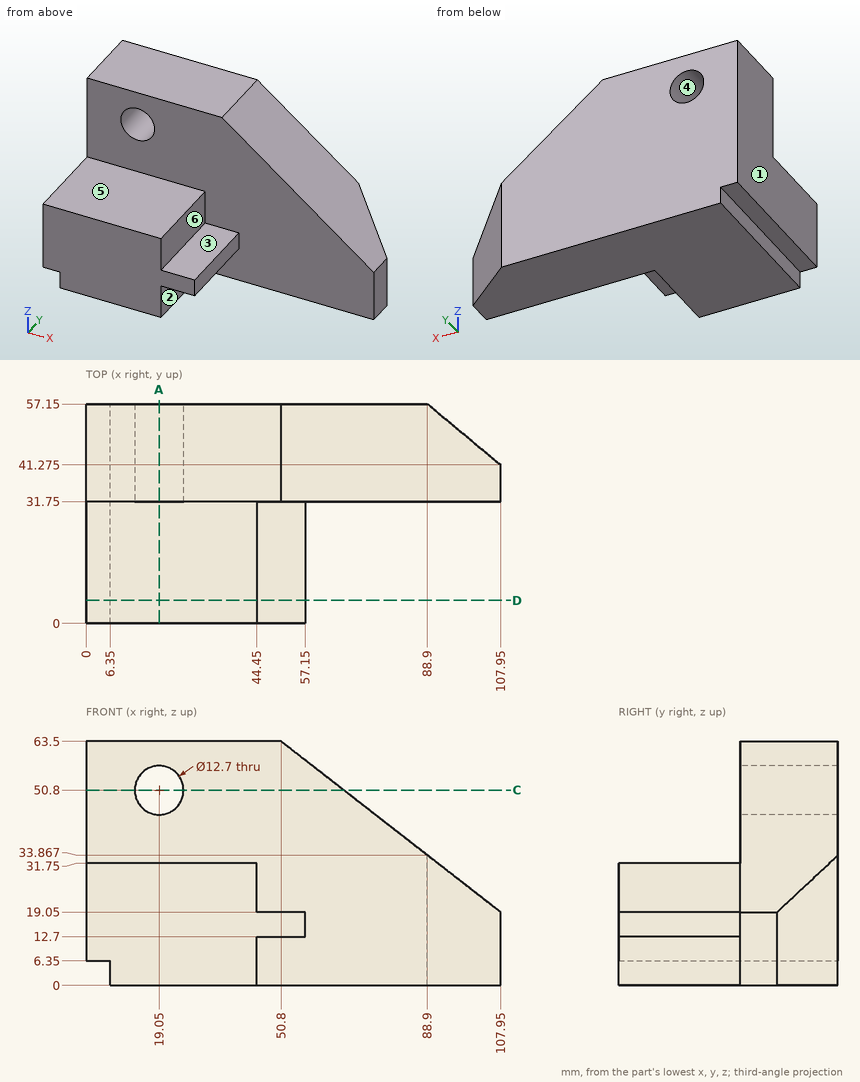
The drawing under review shows one solid part. Ordinate dimensions are in mm from its lowest x, y, z. A direction names the side the tool comes from. Give positions to 0.01 mm unless a question says otherwise; leave off trailing zeros. Write each loop counter-clockwise with the first axis right and the second up, starting at its lowest first coordinate (ties: lowest second). Pieces come first, ordered by that corner, then holes.
1. Add section C-C, the plane z = 50.8. Write out the cut boundary in (x, y), plus the area to 3 significant figures.
2. Add section A-A, the plane x = 19.05. Write out the cut boundary in (y, z), plus the area to 3 significant figures.
3. For P1, Ø14, axis at x = 52, y = 18.5, coming from the -Z side; P2, Ø1.9, axis at x = 2, y = 21, coming from the -Z side; P3, Ø1.5, axis at x = 53.5, y = 12.5, coming from the +Z side, all flat-tipped, find the tip position at first contact; note any pin that passes through.
4. Wall thickness on L1, parallel to Z at x = 19, y = 46; L2, parallel to Y at x = 31, z = 53; L3, parallel to X at y = 11, z = 24: over which ranges is each line inside the solid? List them lowest first.
5. Tool access review of the marked faces 1, 2 and 3: name each direction out of +Z, -Z, +X, -X, +Y, -Y from which nothing blocks a thin tool from reaching the whole face with its end or side.
6. Add section D-D, the plane y = 6. Write out the cut boundary in (x, z).
7. Draft analysis for pull direction X (two halves, no side actions). For the marked faces 4, 5 and 6, state which applies: +X half, -X half, draft (parallel to the pull), parting line (faces both ways), or undercut.
Worked answers:
1. outline: (0, 31.75) - (12.7, 31.75) - (12.7, 57.15) - (0, 57.15) - close; (25.4, 31.75) - (67.13, 31.75) - (67.13, 57.15) - (25.4, 57.15) - close
1. area: 1,380 mm2
2. outline: (0, 0) - (57.15, 0) - (57.15, 44.45) - (31.75, 44.45) - (31.75, 31.75) - (0, 31.75) - close; (31.75, 57.15) - (57.15, 57.15) - (57.15, 63.5) - (31.75, 63.5) - close
2. area: 2,300 mm2
3. P1: stops at z = 12.7
3. P2: stops at z = 6.35
3. P3: stops at z = 19.05
4. L1: z = 0 to 44.45, 57.15 to 63.5
4. L2: y = 31.75 to 57.15
4. L3: x = 0 to 44.45
5. face 1: +Z, -Z, -X, +Y, -Y
5. face 2: -Z, +X, -Y
5. face 3: +Z, +X, -Y
6. outline: (0, 6.35) - (6.35, 6.35) - (6.35, 0) - (44.45, 0) - (44.45, 12.7) - (57.15, 12.7) - (57.15, 19.05) - (44.45, 19.05) - (44.45, 31.75) - (0, 31.75) - close
7. face 4: undercut
7. face 5: draft
7. face 6: +X half
